Geometry check sheet. Reference: drawing and pictorial views, mm from the part's lowest x, y, z. Coordinates: 2 decimals unless noted, no trailing zeros. Loops run counter-clockwise (first coordinate to the right, second up) from the corner with the lowest first, then second, coordinate; pieces in that order, holes last. Notation, with made-up numbers: (76, 35.25) - (100, 35.25) arc R17 cw to (100, 40.25) - close; hole circle Ø4 at (18.5, -32.5). An arc over 180 degrees is marked (long way). One line per item, written item: value.
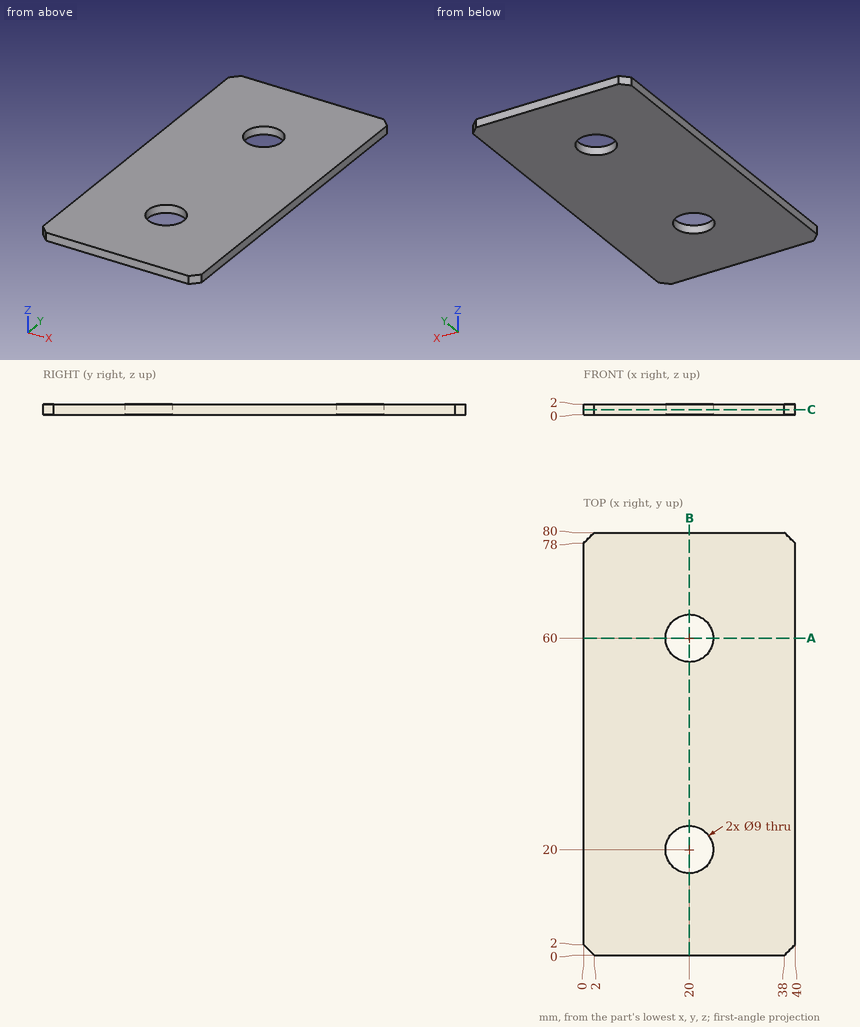
(1) Cross-section at C-C on z = 0.95. Record the cut outline in (x, y), and give its area (3 significant figures).
Reply:
outline: (0, 2) - (2, 0) - (38, 0) - (40, 2) - (40, 78) - (38, 80) - (2, 80) - (0, 78) - close; hole circle Ø9 at (20, 20); hole circle Ø9 at (20, 60)
area: 3,060 mm2
(2) Material ranges on probe 1 along Y at (x, z) = (20, 0.9); probe 2 along Y at (x, z) = (21, 0.55), recorded low to high. Write a range as from..to.
Reply:
probe 1: 0..15.5, 24.5..55.5, 64.5..80
probe 2: 0..15.61, 24.39..55.61, 64.39..80
(3) Cross-section at A-A on y = 60. Record the cut outline in (x, z).
Reply:
outline: (0, 0) - (15.5, 0) - (15.5, 2) - (0, 2) - close; (24.5, 0) - (40, 0) - (40, 2) - (24.5, 2) - close
(4) Go/stop test with a flat-tipped pin: pin 1 Ø10.5 at (x, y) = (20, 20) entering from +Z. Record where the tip stops, or that it passes through.
Reply:
pin 1: z = 2
(5) Cross-section at B-B on x = 20. Record the cut outline in (y, z), and give its area (3 significant figures).
Reply:
outline: (0, 0) - (15.5, 0) - (15.5, 2) - (0, 2) - close; (24.5, 0) - (55.5, 0) - (55.5, 2) - (24.5, 2) - close; (64.5, 0) - (80, 0) - (80, 2) - (64.5, 2) - close
area: 124 mm2
